Geometry check sheet. Reference: the model listing, model coordinates, mm. A direction names the side the tool comes from. Coordinates: 2 decimals unless noted, no trailing zeros. Write each loop counter-clockwise with the first axis right and the second up, starting at its lowest first coordinate (ties: lowest second). Pieces come first, ordered by that corner, then holes. Notation, with made-up numbers: M -13,86 L 2,86 A11 ccw 2,103 Z; hole C -12.5,35 d3. An arc over 180 degrees is marked long. Put each result on its own line as item: value. Start each with the question number.
1) Cross-section at D-D on z = -9. Record the cut outline in (x, y).
2) Cross-section at C-C on y = 41. Record the cut outline in (x, z), plus the area to 3 significant figures.
3) Cross-section at B-B on x = 92.5. Record the cut outline in (y, z), plus the area to 3 significant figures.
4) Scan lines: line 1 along X through (y, z) = (4.5, 0); line 2 along X through (y, z) = (39, -8); line 3 along X through (y, z) = (28.5, 18). Record each from-to range of solid material in increasing order.
5) Mould release check, pull along Z, two halves, no side actions. Record for faces 4 (the flat face through (80, 5, 15)), 5 (the flat face through (70, 36, 5)), 6 (the cylindrical face through (85.12, 4.93, -1.08)): released by +Z, released by -Z, zero draft, split by the parting line, or undercut.
6) Gauge pin test, flat ends, axial feed: pin 1 (20 mm diameter, centred on y = 26.5, z = 6.5, fed in from -X); pin 2 (16 mm diameter, centred on x = 90, z = 0, fed in from +Y); pin 3 (1 mm diameter, centred on x = 46, y = 28, fed in from -Z). Record the tip position at first contact, or that the pin passes through.
7) Cross-section at A-A on z = 0. Record the cut outline in (x, y), plus the area to 3 significant figures.
8) Set-up check for faces 1 (the flat face through (45, 35, 0)), 2 (the flat face through (10, 5, 15)), 3 (the flat face through (83, 10, 0)): record each of +Z, -Z, +X, -X, +Y, -Y from which the full face is reachable in a straight line by a thin tool's end or side.
from build123d import *

# Parameters (mm, degrees)
SKETCH1_R           = 5
BOSS_EXTRUDE4_DEPTH = 10
BOSS_EXTRUDE6_DEPTH = 60
BOSS_EXTRUDE7_DEPTH = 30


with BuildPart() as part:
    # Sketch1 → Boss-Extrude4 (new body)
    with BuildSketch(Plane(origin=(0, 0, 0), x_dir=(1, 0, 0), z_dir=(0, 1, 0))):
        with BuildLine():
            Line((0, -15), (20, -15))
            Line((20, -15), (20, -25))
            Line((20, -25), (70, -25))
            Line((70, -25), (70, -15))
            Line((70, -15), (90, -15))
            ThreePointArc((90, -15), (105, 0), (90, 15))
            Line((90, 15), (0, 15))
            ThreePointArc((0, 15), (-15, 0), (0, -15))
        make_face()
        with Locations(Location((0, 0, 0), (0, 0, 270))):
            Circle(SKETCH1_R, mode=Mode.SUBTRACT)
        with Locations(Location((90, 0, 0), (0, 0, 270))):
            Circle(SKETCH1_R, mode=Mode.SUBTRACT)
    extrude(amount=BOSS_EXTRUDE4_DEPTH)

    # Sketch4 → Boss-Extrude6 (add)
    with BuildSketch(Plane.XZ):
        Polygon((20, -15), (30, -15), (30, 15), (60, 15), (60, -15), (70, -15), (70, 25), (20, 25), align=None)
    extrude(amount=-BOSS_EXTRUDE6_DEPTH)

    # Sketch5 → Boss-Extrude7 (add)
    with BuildSketch(Plane.ZY.offset(-60)):
        Polygon((-15, 10), (15, 60), (15, 10), align=None)
    extrude(amount=BOSS_EXTRUDE7_DEPTH)


solid = part.part
Answer key:
1. outline: M -12,0 L 102,0 L 102,10 L 70,10 L 70,60 L 60,60 L 60,20 L 30,20 L 30,60 L 20,60 L 20,10 L -12,10 Z
2. outline: M 20,-15 L 30,-15 L 30,3.6 L 60,3.6 L 60,-15 L 70,-15 L 70,25 L 20,25 Z
2. area: 1,440 mm²
3. outline: M 0,-14.79 L 10,-14.79 L 10,-4.33 L 0,-4.33 Z; M 0,4.33 L 10,4.33 L 10,14.79 L 0,14.79 Z
3. area: 209 mm²
4. line 1: x = -15 to -5, 5 to 85, 95 to 105
4. line 2: x = 20 to 30, 60 to 70
4. line 3: x = 20 to 70
5. face 4: released by +Z
5. face 5: zero draft
5. face 6: undercut
6. pin 1: stops at x = 20
6. pin 2: stops at y = 10
6. pin 3: stops at z = -4.5
7. outline: M -15,0 L -5,0 L -5,10 L -15,10 Z; M 5,0 L 85,0 L 85,10 L 70,10 L 70,60 L 60,60 L 60,35 L 30,35 L 30,60 L 20,60 L 20,10 L 5,10 Z; M 95,0 L 105,0 L 105,10 L 95,10 Z
7. area: 2,750 mm²
8. face 1: -Z, +Y
8. face 2: +Z, -X, +Y, -Y
8. face 3: +Z, -Z, +X, +Y
